```python
from build123d import *

# Parameters (mm, degrees)
SKETCH003_W     = 43.18
SKETCH003_H     = 17.8
PAD002_DEPTH    = 1.6
SKETCH004_W     = 9.25
SKETCH004_H     = 7.7
PAD003_DEPTH    = 3.9
SKETCH005_R     = 0.925
POCKET001_DEPTH = 5


with BuildPart() as part:
    # Sketch003 → Pad002 (new body)
    with BuildSketch(Plane.XZ):
        with Locations((21.59, 8.9)):
            Rectangle(SKETCH003_W, SKETCH003_H)
    extrude(amount=PAD002_DEPTH)

    # Sketch004 (on Face5 of Pad002) → Pad003 (join)
    with BuildSketch(Plane(origin=(0, 0, 0), x_dir=(1, 0, 0), z_dir=(0, 1, 0))):
        with Locations((3.175, -8.9)):
            Rectangle(SKETCH004_W, SKETCH004_H)
    extrude(amount=PAD003_DEPTH)

    # Sketch005 (on Face4 of Pad003) → Pocket001 (cut)
    with BuildSketch(Plane(origin=(0, 0, 0), x_dir=(1, 0, 0), z_dir=(0, 1, 0))):
        with Locations((1.27, -16.52)):
            Circle(SKETCH005_R)
        with Locations((1.27, -1.28)):
            Circle(SKETCH005_R)
        with Locations((41.91, -1.28)):
            Circle(SKETCH005_R)
        with Locations((41.91, -16.52)):
            Circle(SKETCH005_R)
    extrude(amount=-POCKET001_DEPTH, mode=Mode.SUBTRACT)


with BuildPart() as part_1:
    # Body001 placement: moved
    add(part.part.moved(Location((41.545216, 94.000009, -81.858885))))


solid = part_1.part
```
Here's how the part is built. I have some questions about the finished solid (model axes, mm). A direction names the side the tool comes from. Coordinates: 2 decimals unless noted, no trailing zeros. Order: outer loops, then holes, each group sorted by start corner. A loop starts at its lowest first (then second) coordinate and runs counter-clockwise, first axis right, second up.
1) Imagine slicing it at D-D on y = 95.05. List the corners of the cut face in (x, z) for me, and give its area (3 significant figures).
2) Which directions (+Z, -Z, +X, -X, +Y, -Y) give clear straight access to the entire face, cutting with the end or side of a thin tool? Please do faces 5 (the face through (45, 96, -76.809)), 6 (the face through (45, 96, -69.109)), 7 (the face through (49.345, 96, -73)), 8 (the face through (41.545, 93, -73)).
3) Imagine slicing it at C-C on x = 48.5. List the corners of the cut face in (y, z) for me, and give its area (3 significant figures).
4) We'd pull the mould along X, two halves only. Please class faces 1 (the face through (84.725, 93, -73)), 2 (the face through (63, 94, -73)), 3 (the face through (43.31, 93.21, -66.12)), 4 (the face through (40.095, 96, -73)): +X half, -X half, draft (parallel to the pull), parting line (faces both ways), or undercut.
5) Will these pins go through, and if not, where does the flat tip stop? pin 1 (2.5 mm diameter, centred on x = 83.46, z = -80.58, fed in from -Y); pin 2 (0.8 mm diameter, centred on y = 93, z = -73, fed in from -X); pin 3 (9 mm diameter, centred on x = 64, z = -69, fed in from +Y); pin 4 (2 mm diameter, centred on x = 44.5, y = 96, fed in from -Z).
6) Imagine slicing it at B-B on z = -74.75. List the corners of the cut face in (x, y) for me.
7) I need wall thicknesses on line 1 (X direction, y = 93.05, z = -65.5); line 2 (X direction, y = 93.55, z = -74.5); line 3 (Z direction, x = 49, y = 94.9). Which ranges of each line are inside material? Lowest first, please.
8) Imagine slicing it at A-A on y = 93. List the corners of the cut face in (x, z) for me (3 decimals), and give its area (3 significant figures).
Response values:
1. outline: (40.1, -76.81) - (49.35, -76.81) - (49.35, -69.11) - (40.1, -69.11) - close
1. area: 71.2 mm2
2. face 5: -Z, +X, -X, +Y
2. face 6: +Z, +X, -X, +Y
2. face 7: +Z, -Z, +X, +Y
2. face 8: +Z, -Z, -X, -Y
3. outline: (92.4, -81.86) - (94, -81.86) - (94, -76.81) - (97.9, -76.81) - (97.9, -69.11) - (94, -69.11) - (94, -64.06) - (92.4, -64.06) - close
3. area: 58.5 mm2
4. face 1: +X half
4. face 2: draft
4. face 3: undercut
4. face 4: -X half
5. pin 1: stops at y = 92.4
5. pin 2: stops at x = 41.55
5. pin 3: stops at y = 94
5. pin 4: stops at z = -76.81
6. outline: (40.1, 94) - (41.55, 94) - (41.55, 92.4) - (84.73, 92.4) - (84.73, 94) - (49.35, 94) - (49.35, 97.9) - (40.1, 97.9) - close
7. line 1: x = 41.55 to 41.9, 43.73 to 82.54, 84.37 to 84.73
7. line 2: x = 41.55 to 84.73
7. line 3: z = -76.81 to -69.11
8. outline: (41.545, -81.859) - (84.725, -81.859) - (84.725, -64.059) - (41.545, -64.059) - close; hole circle Ø1.85 at (42.815, -80.579); hole circle Ø1.85 at (42.815, -65.339); hole circle Ø1.85 at (83.455, -80.579); hole circle Ø1.85 at (83.455, -65.339)
8. area: 758 mm2
